Autodesk Fusion 360 part; units mm, degrees
sketch "Sketch1" plane through (0, 0, 0) normal (0, 0, 1) x (1, 0, 0)
  line L0 (7.5, -25) -> (-7.5, -25)
  line L1 (-7.5, -25) -> (-7.5, 25)
  line L2 (7.5, 25) -> (7.5, -25)
  line L3 (7.5, -25) -> (-7.5, 25) construction
  line L4 (-7.5, -25) -> (7.5, 25) construction
  line L5 (-72.5, 25) -> (-72.5, 35)
  line L6 (-72.5, 35) -> (7.5, 35)
  line L7 (7.5, 35) -> (7.5, 25)
  line L8 (-72.5, 25) -> (-7.5, 25)
  circle A0 centre (-0.5, -19) radius 2.1
  circle A1 centre (-0.5, -9) radius 2.1
  dimension "d1" = 50
  dimension "d2" = 15
  dimension "d3" = 10
  dimension "d4" = 80
  dimension "d11" = 4.2
  dimension "d12" = 4.2
  dimension "d13" = 6
  dimension "d14" = 10
  dimension "d15" = 8
  dimension "d16" = 8
  dimension "d19" = 7
extrude "Extrude1" add sketch "Sketch1" along normal blind 14
sketch "Sketch2" plane through (-7.5, 0, 0) normal (-1, 0, 0) x (0, -1, 0)
  line L0 (-25, 0) -> (25, 0)
  line L1 (25, 0) -> (25, 14)
  line L2 (25, 14) -> (-25, 14)
  line L3 (-25, 14) -> (-25, 0)
  line L4 (25, 12.1) -> (4.8, 12.1)
  line L5 (4.8, 12.1) -> (4.8, 1.9)
  line L6 (4.8, 1.9) -> (25, 1.9)
  line L7 (25, 1.9) -> (25, 12.1)
  line L8 (25, 14) -> (-25, 0) construction
  line L9 (-25, 14) -> (25, 0) construction
  line L10 (0, 7) -> (45, 7) construction
  dimension "d7" = 10.2
  dimension "d8" = 20.2
extrude "Extrude2" cut sketch "Sketch2" against normal blind 13 contours L1 L4 L5 L6 L7
sketch "Sketch3" plane through (0, 35, 0) normal (0, 1, 0) x (-1, 0, 0)
  line L0 (-7.5, 0) -> (72.5, 0)
  line L1 (72.5, 0) -> (72.5, 14)
  line L2 (72.5, 14) -> (-7.5, 14)
  line L3 (-7.5, 14) -> (-7.5, 0)
fillet "Fillet1" radius 15 1 edges at (7.5, 35, 7)
fillet "Fillet1" radius 7.5 1 edges at (-7.5, 25, 7)
sketch "Sketch4" plane through (0, 35, 0) normal (0, 1, 0) x (-1, 0, 0)
  line L0 (59.5, 14) -> (59.5, 0) construction
  line L1 (7.5, 14) -> (7.5, 0)
  line L2 (7.5, 0) -> (72.5, 0)
  line L3 (72.5, 0) -> (72.5, 14)
  line L4 (72.5, 14) -> (7.5, 14)
  line L5 (72.5, 7) -> (1.5224, 7) construction
  circle A0 centre (59.5, 7) radius 6
  circle A1 centre (42.55, 7) radius 2.75
  circle A2 centre (76.45, 7) radius 2.75
  line L6 (39.8, 7) -> (39.8, 0) construction
  line L7 (79.2, 7) -> (79.2, 0) construction
  circle A3 centre (59.5, 7) radius 1.6
  circle A4 centre (59.5, 7) radius 5.25
  line L8 (42.1444, 9.7199) -> (58.7257, 12.1926)
  line L9 (42.1444, 4.2801) -> (58.7257, 1.8074)
  line L10 (76.8556, 4.2801) -> (60.2743, 1.8074)
  line L11 (76.8556, 9.7199) -> (60.2743, 12.1926)
  point P0 (-7.5, 14)
  dimension "d20" = 67
  dimension "d21" = 12
  dimension "d22" = 5.5
  dimension "d23" = 5.5
  dimension "d24" = 19.7
  dimension "d25" = 19.7
  dimension "d26" = 3.2
  dimension "d31" = 10.5
extrude "Extrude3" cut sketch "Sketch4" against normal blind 5 contours L3 A2 L10 L11 | L3 A0 L10 L11 | A2 | A0 A4 L8 L11 | A0 A4 L10 L11 | A0 A4 L9 L10 | A0 A4 L8 L9 | A0 A1 L8 L9 | A4 | A1
extrude "Extrude4" cut 1 faces at (-60.4127, 35, 7.0214) along direction (0, -1, 0) through all
ref_plane "WorkPlane1" through (-33.5, 0, 7) normal (1, 0, 0) x (0, 1, 0)
split "Split1" [suppressed]
CAD build for the part. Positions are in the model's coordinates, mm. A direction names the side the tool comes from. Coordinates: 2 decimals unless noted, no trailing zeros. Write each loop counter-clockwise with the first axis right and the second up, starting at its lowest first coordinate (ties: lowest second). Pieces come first, ordered by that corner, then holes.
(1) Cut at D-D, the plane x = -54. List the corners of the cut face in (y, z).
(2) Two-plate mould, pull along X, no slides. Class faces 5 (the face through (-48.903, 32.535, 10.728)), 6 (the face through (-39.8, 32.5, 7.1)), 7 (the face through (7.5, -2, 7)), 8 (the face through (-1, -4.8, 7)): +X half, -X half, draft (parallel to the pull), parting line (faces both ways), or undercut.
(3) Cut at C-C, the plane x = -0.5. List the corners of the cut face in (y, z), and give its area (3 significant figures).
(4) Cut at B-B, the plane y = -9. List the corners of the cut face in (x, z).
(5) Drill centre lines: probe 1 along X at (y, z) = (-19, 0.5); probe 2 along Z at (x, y) = (-59.5, 28.15); probe 3 along Y at (x, z) = (-67, 6.75). Where is each one in solid material? Low to high.
(6) Flat gauge pins, fed straight in: pin 1 (4 mm diameter, centred on x = -0.5, y = -9, fed in from -Z); pin 2 (4 mm diameter, centred on x = -36, z = 5.5, fed in from -Y); pin 3 (7 mm diameter, centred on y = -13.5, z = 10.5, fed in from -X). Where does each tip first touch, or does it go through?
(7) Cut at A-A, the plane z = 7. List the corners of the cut face in (x, y).
(8) 3-axis set-ups, long thin cutter, end or side, ignore diameter. For faces 1 (the face through (6, -25, 7)), 2 (the face through (-1, -15, 1.9)), 3 (the face through (-59.6, 32.5, 13)), 4 (the face through (-7.5, 1, 7)): which of +Z, -Z, +X, -X, +Y, -Y reach the whole face in a straight line?
Geometry says:
1. outline: (25, 0) - (35, 0) - (35, 2.51) - (30, 2.51) - (30, 11.49) - (35, 11.49) - (35, 14) - (25, 14) - close
2. face 5: undercut
2. face 6: -X half
2. face 7: +X half
2. face 8: draft
3. outline: (-25, 0) - (-21.1, 0) - (-21.1, 1.9) - (-25, 1.9) - close; (-25, 12.1) - (-21.1, 12.1) - (-21.1, 14) - (-25, 14) - close; (-16.9, 0) - (-11.1, 0) - (-11.1, 1.9) - (-16.9, 1.9) - close; (-16.9, 12.1) - (-11.1, 12.1) - (-11.1, 14) - (-16.9, 14) - close; (-6.9, 0) - (33.27, 0) - (33.27, 14) - (-6.9, 14) - (-6.9, 12.1) - (-4.8, 12.1) - (-4.8, 1.9) - (-6.9, 1.9) - close
3. area: 578 mm2
4. outline: (-7.5, 0) - (-2.6, 0) - (-2.6, 1.9) - (-7.5, 1.9) - close; (-7.5, 12.1) - (-2.6, 12.1) - (-2.6, 14) - (-7.5, 14) - close; (1.6, 0) - (7.5, 0) - (7.5, 14) - (1.6, 14) - (1.6, 12.1) - (5.5, 12.1) - (5.5, 1.9) - (1.6, 1.9) - close
5. probe 1: x = -7.5 to -2.6, 1.6 to 7.5
5. probe 2: z = 0 to 5.4, 8.6 to 14
5. probe 3: y = 25 to 30
6. pin 1: passes through
6. pin 2: stops at y = 25
6. pin 3: stops at x = -7.5
7. outline: (-72.5, 25) - (-61.1, 25) - (-61.1, 30) - (-72.5, 30) - close; (-57.9, 25) - (-15, 25) arc R7.5 cw to (-7.5, 17.5) - (-7.5, -4.8) - (5.5, -4.8) - (5.5, -25) - (7.5, -25) - (7.5, 20) arc R15 ccw to (-7.5, 35) - (-39.8, 35) - (-39.8, 30) - (-57.9, 30) - close
8. face 1: +Z, -Z, +X, -X, -Y
8. face 2: -X, -Y
8. face 3: +Y
8. face 4: +Z, -Z, -X, -Y
